Check sheet for the modelled part. Datum: model origin and axes. Units: mm. Face numbers are marked on the shaded views. A direction names the side the tool comes from. Round coordinates to 2 decimals unless told otherwise and drop trailing zeros. Write each loop counter-clockwise with the first axis right and the second up, starting at its lowest first coordinate (ties: lowest second). Pieces come first, ordered by that corner, then holes.
Item 1: Section check D-D, the plane x = 85. Record the cut outline in (y, z).
Item 2: Set-up check for the marked faces 1 and 2: record each of +Z, -Z, +X, -X, +Y, -Y from which the full face is reachable in a straight line by a thin tool's end or side.
Item 3: Material ranges on line 1 along Y through (x, z) = (35.5, -62.5); line 2 along Z through (x, y) = (-6.5, -23.5); line 3 along X through (y, z) = (-8, -3.5), recorded low to high.
Item 4: Depth check by flat-ended pin: pin 1 (2.5 mm diameter, centred on x = -32.5, y = -7.5, fed in from +Z); pin 2 (4 mm diameter, centred on x = -0.5, y = -13, fed in from +Z); pin 3 (1.5 mm diameter, centred on x = 97.5, y = -17.5, fed in from -Z); pin 4 (3 mm diameter, centred on y = -3, z = -54, fed in from +X). Enter the tip coordinate at first touch or a pass-through.
Item 5: Section check B-B, the plane x = 0. Record the cut outline in (y, z).
Item 6: Section check C-C, the plane z = 48. Record the cut outline in (x, y).
Item 7: Section check A-A, the plane y = -5. Record the cut outline in (x, z).
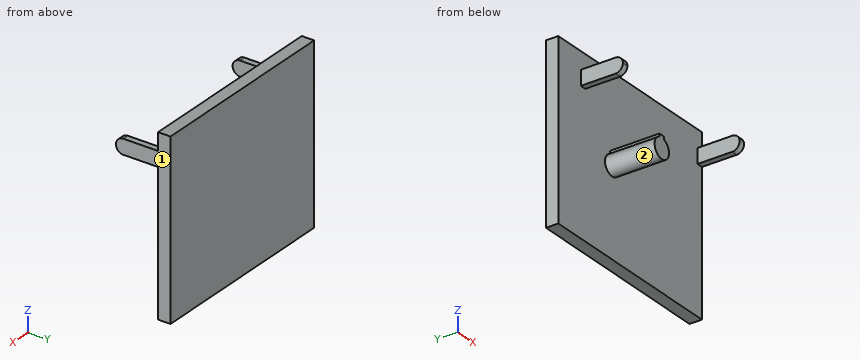
from build123d import *

# Parameters (mm, degrees)
F0_W     = 160
F0_H     = 140
F1_DEPTH = 10
F3_DEPTH = 40
F5_DEPTH = 5
F8_DEPTH = 5


with BuildPart() as f1:
    # F0 (on Front) → F1 (new body)
    with BuildSketch(Plane.XZ):
        with Locations((20, 0)):
            Rectangle(F0_W, F0_H)
    extrude(amount=-F1_DEPTH)

    # F2 (on face) → F3 (join)
    with BuildSketch(Plane.XZ):
        with BuildLine():
            Line((-2.5, 10), (-2.5, 7.5993420768))
            ThreePointArc((-2.5, 7.5993420768), (0, -8), (2.5, 7.5993420768))
            Line((2.5, 7.5993420768), (2.5, 10))
            Line((2.5, 10), (-2.5, 10))
        make_face()
    extrude(amount=F3_DEPTH)

    # F4 (on face) → F5 (join)
    with BuildSketch(Plane.YZ.offset(100)):
        with BuildLine():
            ThreePointArc((-28, 56), (-34, 50), (-28, 44))
            Line((-28, 44), (10, 44))
            Line((10, 44), (10, 56))
            Line((10, 56), (-28, 56))
        make_face()
    extrude(amount=-F5_DEPTH)

    # F7 (on offset) → F8 (join)
    with BuildSketch(Plane.YZ.offset(-35)):
        with BuildLine():
            Line((10, 56), (-28, 56))
            ThreePointArc((-28, 56), (-32.2426406871, 54.2426406871), (-34, 50))
            Line((-34, 50), (10, 50))
            Line((10, 50), (10, 56))
        make_face()
        with BuildLine():
            Line((10, 50), (-34, 50))
            ThreePointArc((-34, 50), (-32.2426406871, 45.7573593129), (-28, 44))
            Line((-28, 44), (10, 44))
            Line((10, 44), (10, 50))
        make_face()
    extrude(amount=F8_DEPTH)


solid = f1.part
Values found:
1. outline: (0, -70) - (10, -70) - (10, 70) - (0, 70) - close
2. face 1: +Z, -Z, +X, +Y, -Y
2. face 2: -Y
3. line 1: y = 0 to 10
3. line 2: z = -4.66 to 4.66
3. line 3: x = -7.19 to 7.19
4. pin 1: stops at z = 56
4. pin 2: stops at z = 10
4. pin 3: stops at z = 44
4. pin 4: passes through
5. outline: (-40, -8) - (0, -8) - (0, -70) - (10, -70) - (10, 70) - (0, 70) - (0, 10) - (-40, 10) - close
6. outline: (-60, 0) - (-35, 0) - (-35, -33.66) - (-30, -33.66) - (-30, 0) - (95, 0) - (95, -33.66) - (100, -33.66) - (100, 10) - (-60, 10) - close
7. outline: (-35, 44) - (-30, 44) - (-30, 56) - (-35, 56) - close; (-2.5, 7.6) arc R8 ccw (long way) to (2.5, 7.6) - (2.5, 10) - (-2.5, 10) - close; (95, 44) - (100, 44) - (100, 56) - (95, 56) - close
